Answer from the drawing. Dimensions are ordinates in mm from the lowest x, y and z of the part. A direction names the side the tool comes from. Give positions to 0.01 mm unless a question says otherwise; leave off trailing zeros. Order: outer loops, then holes, each group sorted by start corner. A loop starts at its lowest first (then second) coordinate and runs counter-clockwise, first axis right, second up. Notation, with made-up numbers: (18, 41.5) -> (69, 41.5) arc R31 ccw to (69, 71.5) -> close; hole circle Ø7 at (58, 34). An arc over 180 degrees is marked (long way). Answer as CSV lines item,"result". Start each with the question number.
1) Find section B-B (y = 13.5). Determine the outline of the cut face in (x, z), and give its area (3 significant figures).
2) The mould has two halves that part along Z. Classify the marked faces 1, 2, 3 and 4: +Z half, -Z half, draft (parallel to the pull), parting line (faces both ways), or undercut.
3) Straight lines are drawn through the part: L1, parallel to Y at x = 27.5, z = 15; L2, parallel to Z at x = 9.75, y = 7.25. For each, find the intervals that lie inside material, in ascending order. Write a range as from..to.
4) Flat-ended cylindrical pins translate along their axes: pin 1 Ø1 at (y, z) = (14.5, 7) entering from -X; pin 2 Ø1 at (x, y) = (7, 8) entering from -Z. Find the tip coordinate at first contact, or state that the pin passes through.
5) Find section D-D (y = 7.25). Determine the outline of the cut face in (x, z).
6) For the marked faces 5 and 6, determine the directions among +Z, -Z, +X, -X, +Y, -Y from which every point of the face is accessible in a straight line to the end or side of a thin tool.
7) Find section A-A (z = 15). Determine the outline of the cut face in (x, y), and give its area (3 significant figures).
8) Find section C-C (x = 15). Determine the outline of the cut face in (y, z).
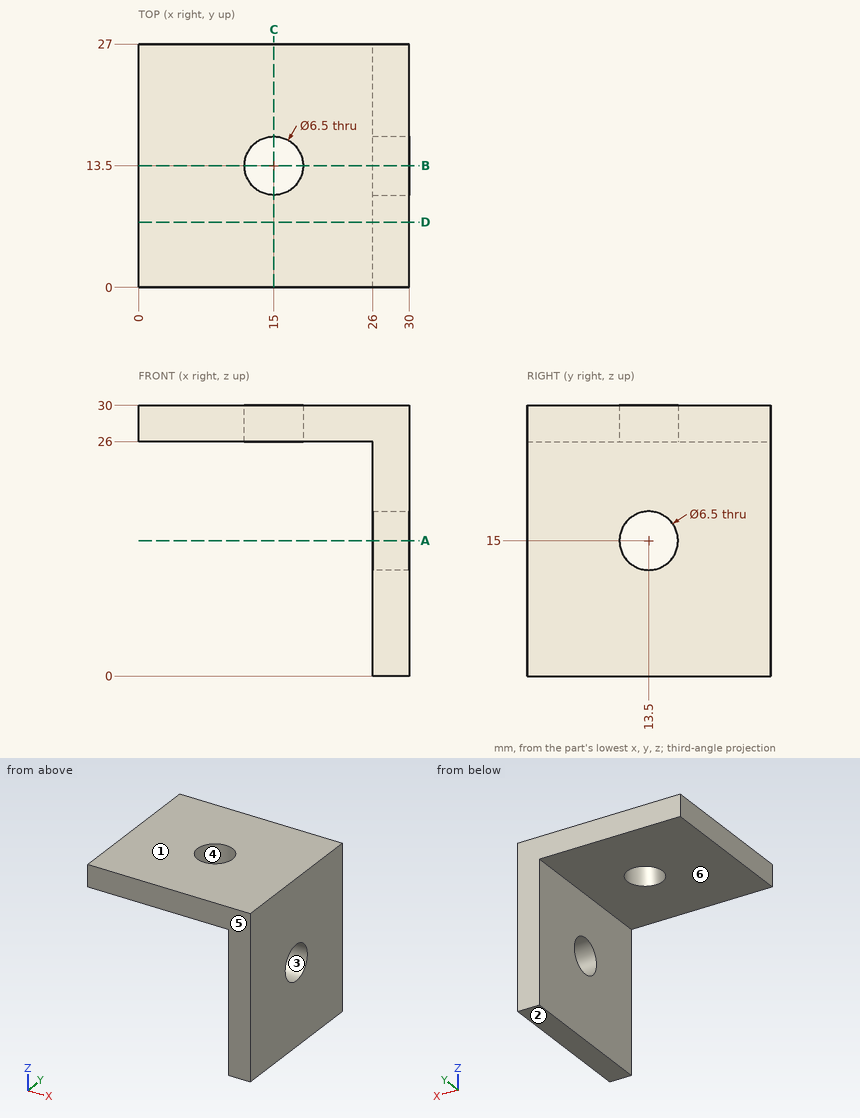
Findings below:
1,outline,"(0, 26) -> (11.75, 26) -> (11.75, 30) -> (0, 30) -> close; (18.25, 26) -> (26, 26) -> (26, 18.25) -> (30, 18.25) -> (30, 30) -> (18.25, 30) -> close; (26, 0) -> (30, 0) -> (30, 11.75) -> (26, 11.75) -> close"
1,area,"172 mm²"
2,face 1,"+Z half"
2,face 2,"-Z half"
2,face 3,"undercut"
2,face 4,"draft"
3,L1,"0..10.25, 16.75..27"
3,L2,"26..30"
4,pin 1,"x = 26"
4,pin 2,"z = 26"
5,outline,"(0, 26) -> (26, 26) -> (26, 0) -> (30, 0) -> (30, 30) -> (0, 30) -> close"
6,face 5,"+Z, -Z, +X, -X, -Y"
6,face 6,"-Z, -X, +Y, -Y"
7,outline,"(26, 0) -> (30, 0) -> (30, 10.25) -> (26, 10.25) -> close; (26, 16.75) -> (30, 16.75) -> (30, 27) -> (26, 27) -> close"
7,area,"82.0 mm²"
8,outline,"(0, 26) -> (10.25, 26) -> (10.25, 30) -> (0, 30) -> close; (16.75, 26) -> (27, 26) -> (27, 30) -> (16.75, 30) -> close"
